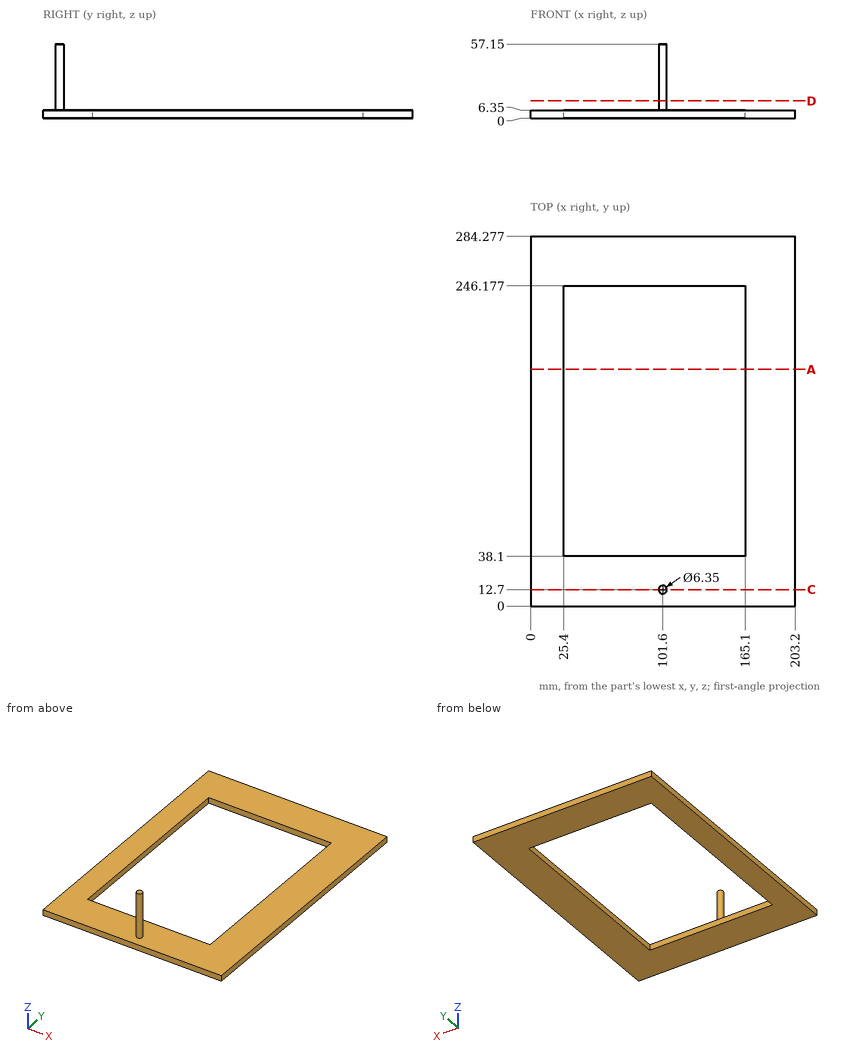
Check sheet for the drawn part. Datum: minimum x, y, z corner. Units: mm. Coordinates: 2 decimals unless noted, no trailing zeros. Write each loop counter-clockwise with the first axis right and the second up, starting at its lowest first coordinate (ties: lowest second). Pieces come first, ordered by that corner, then holes. Notation, with made-up numbers: (61.5, 81.5) - (117.5, 81.5) arc R18 ccw to (117.5, 93.5) - close; hole circle Ø9 at (-28.75, 63). An arc over 180 degrees is marked (long way). Answer as a JSON object with one key per item and string values.
(1) Cross-section at C-C on y = 12.7. Record the cut outline in (x, z) (3 decimals).
Report:
{"outline": "(0, 0) - (203.2, 0) - (203.2, 6.35) - (104.775, 6.35) - (104.775, 57.15) - (98.425, 57.15) - (98.425, 6.35) - (0, 6.35) - close"}
(2) Cross-section at A-A on y = 182. Record the cut outline in (x, z), plus the area to 3 significant figures.
Report:
{"outline": "(0, 0) - (25.4, 0) - (25.4, 6.35) - (0, 6.35) - close; (165.1, 0) - (203.2, 0) - (203.2, 6.35) - (165.1, 6.35) - close", "area": "403 mm^2"}
(3) Cross-section at D-D on z = 13.5. Record the cut outline in (x, y) (3 decimals).
Report:
{"outline": "circle Ø6.35 at (101.6, 12.7)"}
(4) Thickness scan on line 1 along Y through (x, z) = (62.5, 3.5); line 2 along X through (y, z) = (88, 5.5); line 3 along Z through (x, y) = (150.5, 251.5). Record the ranges inside material, lowest first.
Report:
{"line 1": "0 to 38.1, 246.18 to 284.28", "line 2": "0 to 25.4, 165.1 to 203.2", "line 3": "0 to 6.35"}
